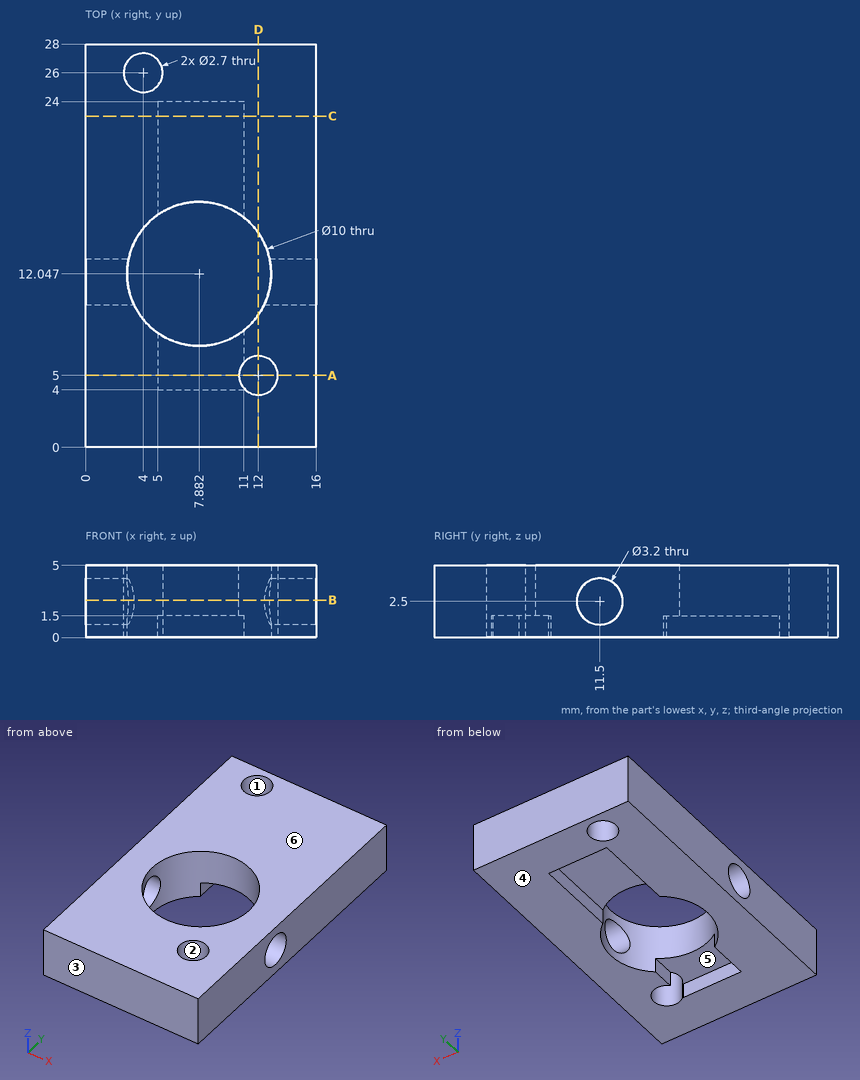
Print and shaded views of the part. All mm, measured from the part's lowest x, y and z. A direction names the side the tool comes from. Round coordinates to 2 decimals unless told otherwise and drop trailing zeros. Write each loop counter-clockwise with the first axis right and the second up, starting at its lowest first coordinate (ties: lowest second). Pieces come first, ordered by that corner, then holes. Notation, with made-up numbers: (20.25, 11) - (76.25, 11) arc R22 cw to (76.25, 36) - close; hole circle Ø5 at (37.5, 16.25). An arc over 180 degrees is marked (long way). Use CSV: the item, a comma, the result in double quotes. Start each with the question number.
Item 1: Band-saw the part on D-D (x = 12). Write the cut outline in (y, z).
Item 2: Band-saw the part on B-B (z = 2.6). State how many separate pieces and enclosed holes the cut face has, and give its area (3 significant figures).
Item 3: Pin check, flat tips, straight feed: P1, Ø3.5, axis at x = 4, y = 26, coming from the +Z side; P2, Ø2, axis at x = 9, y = 6.5, coming from the -Z side. Stop position of each tip, or through.
Item 4: Band-saw the part on A-A (y = 5). Write the cut outline in (x, z).
Item 5: Tool access for the marked faces 5 and 6: list every direction of +Z, -Z, +X, -X, +Y, -Y with a clear straight run to the whole face (end or side of a thin tool).
Item 6: Drill centre lines: L1, parallel to Z at x = 14.15, y = 11.5; L2, parallel to X at y = 7, z = 1.3; L3, parallel to Y at x = 11.5, z = 3.2 (1 decimal). Where is each one in solid material? Low to high. Write a range as [from, to].
Item 7: Band-saw the part on C-C (y = 23). Write the cut outline in (x, z), and give its area (3 significant figures).
Item 8: Two-plate mould, pull along Y, no slides. Class the marked faces 1, 2, 3 and 4: released by +Y, released by -Y, zero draft, split by the parting line, or undercut.
Checked values:
1,outline,"(0, 0) - (3.65, 0) - (3.65, 5) - (0, 5) - close; (6.35, 0) - (9.21, 0) - (9.21, 5) - (6.35, 5) - close; (14.88, 0) - (28, 0) - (28, 5) - (14.88, 5) - close"
2,separate pieces,"2"
2,enclosed holes,"2"
2,area,"338 mm²"
3,P1,"stops at z = 5"
3,P2,"stops at z = 1.5"
4,outline,"(0, 0) - (5, 0) - (5, 1.5) - (10.65, 1.5) - (10.65, 5) - (0, 5) - close; (13.35, 0) - (16, 0) - (16, 5) - (13.35, 5) - close"
5,face 5,"-Z"
5,face 6,"+Z, +X, -X, +Y, -Y"
6,L1,"z = [0, 0.9], [4.1, 5]"
6,L2,"x = [0, 5], [11, 16]"
6,L3,"y = [0, 3.7], [6.3, 8.6], [15.5, 28]"
7,outline,"(0, 0) - (5, 0) - (5, 1.5) - (11, 1.5) - (11, 0) - (16, 0) - (16, 5) - (0, 5) - close"
7,area,"71.0 mm²"
8,face 1,"undercut"
8,face 2,"undercut"
8,face 3,"released by -Y"
8,face 4,"zero draft"
